Read the model definition and answer for the solid it produces. Units are mm, in the model's axes. A direction names the side the tool comes from. Coordinates: 2 decimals unless noted, no trailing zeros. Order: outer loops, then holes, each group sorted by start corner. A loop starts at its lowest first (then second) coordinate and runs counter-clockwise, first axis right, second up. Notation, with made-up numbers: M -36,35.5 L -2,35.5 A26 ccw -2,72.5 Z; hole C -18,71 d4. An arc over 180 degrees is marked long. Use a Markdown table: item, result. Add a question column.
1) Each of these flat-tipped pins is pushed along its axis until it touches: pin 1 Ø4 at (x, y) = (-45, 32) entering from -Z; pin 2 Ø8 at (x, z) = (-17.5, 23.5) entering from +Y; pin 3 Ø10.5 at (x, z) = (-54, 13.5) entering from -Y. Where does it stop, or does it pass through?
2) Find section D-D on x = -55.5. Write down the section's boundary in (y, z).
3) Find the intervals of material crossed by probe 1 along Z at (x, y) = (-55.5, 41); probe 2 along X at (y, z) = (51, -15); probe 3 along X at (y, z) = (13, 17), in increasing order. Write a range as [from, to].
4) Find section C-C on z = 15. Write down the section's boundary in (x, y), plus the area to 3 significant figures.
5) Find section A-A on z = -8. Write down the section's boundary in (x, y), plus the area to 3 significant figures.
6) The mould has two halves that part along Z. Classify faces 6 (the face through (-40.5, 29.8, 0.6)), 7 (the face through (-59.5, 55.4, 18)), 8 (the face through (-58, 55, 30)): released by +Z, released by -Z, zero draft, split by the parting line, or undercut.
7) For faces 1 (the face through (-58, 55, -30)), 2 (the face through (-65.5, 35, 0)), 3 (the face through (-70.5, 78, 0)), 4 (the face through (-69, 74, -10)), 5 (the face through (-58, 80, 0)), determine the directions among +Z, -Z, +X, -X, +Y, -Y from which every point of the face is accessible in a straight line to the end or side of a thin tool.
8) Find section B-B on y = 54. Write down the section's boundary in (x, z).
from build123d import *

# Parameters (mm, degrees)
SKETCH1_W           = 81
SKETCH1_H           = 81
BOSS_EXTRUDE1_DEPTH = 10
BOSS_EXTRUDE2_START = 10
SKETCH2_W           = 3
SKETCH2_H           = 81
BOSS_EXTRUDE2_DEPTH = 100
SKETCH3_W           = 60
SKETCH3_H           = 50
BOSS_EXTRUDE3_DEPTH = 35
CUT_EXTRUDE1_REACH  = 82
SKETCH4_R           = 5
CUT_EXTRUDE4_START  = -20
CUT_EXTRUDE4_DEPTH  = 20


with BuildPart() as part:
    # Sketch1 → Boss-Extrude1 (new body)
    with BuildSketch(Plane(origin=(0, 0, 0), x_dir=(1, 0, 0), z_dir=(0, 1, 0))):
        Rectangle(SKETCH1_W, SKETCH1_H)
    extrude(amount=BOSS_EXTRUDE1_DEPTH)

    # Sketch2 → Boss-Extrude2 (add)
    with BuildSketch(Plane(origin=(0, 0, 0), x_dir=(1, 0, 0), z_dir=(0, 1, 0)).offset(BOSS_EXTRUDE2_START)):
        with Locations((-39, 0)):
            Rectangle(SKETCH2_W, SKETCH2_H)
    extrude(amount=BOSS_EXTRUDE2_DEPTH)

    # Sketch3 → Boss-Extrude3 (add)
    with BuildSketch(Plane.ZY.offset(40.5)):
        with Locations((0, 55)):
            Rectangle(SKETCH3_W, SKETCH3_H)
    extrude(amount=BOSS_EXTRUDE3_DEPTH)

    # Sketch4 → Cut-Extrude1 (cut, up to next)
    with BuildSketch(Plane(origin=(0, 80, 0), x_dir=(1, 0, 0), z_dir=(0, 1, 0)), mode=Mode.PRIVATE) as cut_extrude1_sk1:
        with Locations((-55.5, 15)):
            Circle(SKETCH4_R)
    cut_extrude1_tool1 = extrude(cut_extrude1_sk1.sketch, amount=-CUT_EXTRUDE1_REACH, mode=Mode.PRIVATE) & part.part
    add(cut_extrude1_tool1.solids().sort_by_distance((-55.5, 80, -15))[0], mode=Mode.SUBTRACT)
    # Sketch4 → Cut-Extrude1 (cut, up to next)
    with BuildSketch(Plane(origin=(0, 80, 0), x_dir=(1, 0, 0), z_dir=(0, 1, 0)), mode=Mode.PRIVATE) as cut_extrude1_sk2:
        with Locations((-55.5, -15)):
            Circle(SKETCH4_R)
    cut_extrude1_tool2 = extrude(cut_extrude1_sk2.sketch, amount=-CUT_EXTRUDE1_REACH, mode=Mode.PRIVATE) & part.part
    add(cut_extrude1_tool2.solids().sort_by_distance((-55.5, 80, 15))[0], mode=Mode.SUBTRACT)

    # Sketch5 → Cut-Extrude4 (cut)
    with BuildSketch(Plane.XY.offset(30).offset(CUT_EXTRUDE4_START)):
        Polygon((-75.5, 75), (-75.5, 70), (-65.5, 70), (-65.5, 80), (-70.5, 80), (-70.5, 75), align=None)
        Polygon((-65.5, 30), (-65.5, 40), (-75.5, 40), (-75.5, 35), (-70.5, 35), (-70.5, 30), align=None)
    extrude(amount=-CUT_EXTRUDE4_DEPTH, mode=Mode.SUBTRACT)


solid = part.part
Check result:
| question | item | result |
|---|---|---|
| 1 | pin 1 | stops at z = -30 |
| 1 | pin 2 | stops at y = 10 |
| 1 | pin 3 | stops at y = 30 |
| 2 | outline | M 30,-30 L 80,-30 L 80,-20 L 30,-20 Z; M 30,-10 L 80,-10 L 80,10 L 30,10 Z; M 30,20 L 80,20 L 80,30 L 30,30 Z |
| 3 | probe 1 | z = [-30, -20], [-10, 10], [20, 30] |
| 3 | probe 2 | x = [-75.5, -60.5], [-50.5, -37.5] |
| 3 | probe 3 | x = [-40.5, -37.5] |
| 4 | outline | M -75.5,30 L -60.5,30 L -60.5,80 L -75.5,80 Z; M -50.5,30 L -40.5,30 L -40.5,0 L 40.5,0 L 40.5,10 L -37.5,10 L -37.5,110 L -40.5,110 L -40.5,80 L -50.5,80 Z |
| 4 | area | 2,360 mm2 |
| 5 | outline | M -75.5,30 L -70.5,30 L -70.5,35 L -75.5,35 Z; M -75.5,40 L -65.5,40 L -65.5,30 L -40.5,30 L -40.5,0 L 40.5,0 L 40.5,10 L -37.5,10 L -37.5,110 L -40.5,110 L -40.5,80 L -65.5,80 L -65.5,70 L -75.5,70 Z; M -75.5,75 L -70.5,75 L -70.5,80 L -75.5,80 Z |
| 5 | area | 2,710 mm2 |
| 6 | face 6 | zero draft |
| 6 | face 7 | undercut |
| 6 | face 8 | released by +Z |
| 7 | face 1 | -Z, -X, +Y, -Y |
| 7 | face 2 | -Y |
| 7 | face 3 | +Y |
| 7 | face 4 | none |
| 7 | face 5 | +Z, -Z, -X, +Y |
| 8 | outline | M -75.5,-30 L -40.5,-30 L -40.5,-40.5 L -37.5,-40.5 L -37.5,40.5 L -40.5,40.5 L -40.5,30 L -75.5,30 Z; hole C -55.5,-15 d10; hole C -55.5,15 d10 |
